Autodesk Inventor part; units mm, degrees
ref_plane "YZ Plane" through (0, 0, 0) normal (1, 0, 0) x (0, 1, 0)
ref_plane "XZ Plane" through (0, 0, 0) normal (0, 1, 0) x (-1, 0, 0)
ref_plane "XY Plane" through (0, 0, 0) normal (0, 0, 1) x (1, 0, 0)
sketch "Sketch1" plane through (0, 0, 0) normal (0, 0, 1) x (1, 0, 0)
  line L0 (0, 0) -> (225, 0)
  line L1 (225, 0) -> (225, 50)
  line L2 (225, 50) -> (0, 50)
  line L3 (0, 50) -> (0, 0)
  line L4 (-3, 45) -> (0, 45)
  line L5 (0, 45) -> (0, 38.75)
  line L6 (0, 38.75) -> (-3, 38.75)
  line L7 (-3, 38.75) -> (-3, 45)
  line L8 (0, 0) -> (15, 0)
  line L9 (15, 0) -> (15, -3)
  line L10 (15, -3) -> (0, -3)
  line L11 (0, -3) -> (0, 0)
  line L12 (-3, 33.75) -> (0, 33.75)
  line L13 (0, 33.75) -> (0, 27.5)
  line L14 (-3, 27.5) -> (-3, 33.75)
  line L15 (0, 27.5) -> (-3, 27.5)
  line L16 (-3, 22.5) -> (0, 22.5)
  line L17 (0, 22.5) -> (0, 16.25)
  line L18 (-3, 16.25) -> (-3, 22.5)
  line L19 (0, 16.25) -> (-3, 16.25)
  line L20 (-3, 11.25) -> (0, 11.25)
  line L21 (0, 11.25) -> (0, 5)
  line L22 (-3, 5) -> (-3, 11.25)
  line L23 (0, 5) -> (-3, 5)
  line L24 (225, 45) -> (228, 45)
  line L25 (228, 45) -> (228, 38.75)
  line L26 (225, 38.75) -> (225, 45)
  line L27 (228, 38.75) -> (225, 38.75)
  line L28 (225, 33.75) -> (228, 33.75)
  line L29 (228, 33.75) -> (228, 27.5)
  line L30 (225, 27.5) -> (225, 33.75)
  line L31 (228, 27.5) -> (225, 27.5)
  line L32 (225, 22.5) -> (228, 22.5)
  line L33 (228, 22.5) -> (228, 16.25)
  line L34 (225, 16.25) -> (225, 22.5)
  line L35 (228, 16.25) -> (225, 16.25)
  line L36 (225, 11.25) -> (228, 11.25)
  line L37 (228, 11.25) -> (228, 5)
  line L38 (225, 5) -> (225, 11.25)
  line L39 (228, 5) -> (225, 5)
  line L40 (45, -3) -> (30, -3)
  line L41 (30, -3) -> (30, 0)
  line L42 (45, 0) -> (45, -3)
  line L43 (30, 0) -> (45, 0)
  line L44 (75, -3) -> (60, -3)
  line L45 (60, -3) -> (60, 0)
  line L46 (75, 0) -> (75, -3)
  line L47 (60, 0) -> (75, 0)
  line L48 (105, -3) -> (90, -3)
  line L49 (90, -3) -> (90, 0)
  line L50 (105, 0) -> (105, -3)
  line L51 (90, 0) -> (105, 0)
  line L52 (135, -3) -> (120, -3)
  line L53 (120, -3) -> (120, 0)
  line L54 (135, 0) -> (135, -3)
  line L55 (120, 0) -> (135, 0)
  line L56 (165, -3) -> (150, -3)
  line L57 (150, -3) -> (150, 0)
  line L58 (165, 0) -> (165, -3)
  line L59 (150, 0) -> (165, 0)
  line L60 (195, -3) -> (180, -3)
  line L61 (180, -3) -> (180, 0)
  line L62 (195, 0) -> (195, -3)
  line L63 (180, 0) -> (195, 0)
  line L64 (225, -3) -> (210, -3)
  line L65 (210, -3) -> (210, 0)
  line L66 (225, 0) -> (225, -3)
  line L67 (210, 0) -> (225, 0)
  line L68 (15, 50) -> (0, 50)
  line L69 (0, 50) -> (0, 53)
  line L70 (15, 53) -> (15, 50)
  line L71 (0, 53) -> (15, 53)
  line L72 (45, 50) -> (30, 50)
  line L73 (30, 50) -> (30, 53)
  line L74 (45, 53) -> (45, 50)
  line L75 (30, 53) -> (45, 53)
  line L76 (75, 50) -> (60, 50)
  line L77 (60, 50) -> (60, 53)
  line L78 (75, 53) -> (75, 50)
  line L79 (60, 53) -> (75, 53)
  line L80 (105, 50) -> (90, 50)
  line L81 (90, 50) -> (90, 53)
  line L82 (105, 53) -> (105, 50)
  line L83 (90, 53) -> (105, 53)
  line L84 (135, 50) -> (120, 50)
  line L85 (120, 50) -> (120, 53)
  line L86 (135, 53) -> (135, 50)
  line L87 (120, 53) -> (135, 53)
  line L88 (165, 50) -> (150, 50)
  line L89 (150, 50) -> (150, 53)
  line L90 (165, 53) -> (165, 50)
  line L91 (150, 53) -> (165, 53)
  line L92 (195, 50) -> (180, 50)
  line L93 (180, 50) -> (180, 53)
  line L94 (195, 53) -> (195, 50)
  line L95 (180, 53) -> (195, 53)
  line L96 (225, 50) -> (210, 50)
  line L97 (210, 50) -> (210, 53)
  line L98 (225, 53) -> (225, 50)
  line L99 (210, 53) -> (225, 53)
  point P0 (0, 38.75)
  point P1 (0, 50)
  dimension "d0" = 225
  dimension "d1" = 50
  dimension "d4" = 6.25
  dimension "d5" = 3
  dimension "d6" = 5
  dimension "d7" = 15
  dimension "d8" = 3
  dimension "d13" = 11.25
  dimension "d16" = 228
  dimension "d21" = 30
  dimension "d24" = 53
extrude "Extrusion1" add sketch "Sketch1" along normal blind 3 contours L3 L2 L1 L0 | L23 L22 L20 L3 | L19 L18 L16 L3 | L15 L14 L12 L3 | L6 L7 L4 L3 | L1 L36 L37 L39 | L1 L32 L33 L35 | L1 L28 L29 L31 | L1 L24 L25 L27
extrude "Extrusion2" add sketch "Sketch1" along normal blind 3 contours L0 L9 L10 L11 | L0 L42 L40 L41 | L0 L46 L44 L45 | L0 L50 L48 L49 | L0 L54 L52 L53 | L69 L71 L70 L2 | L0 L58 L56 L57 | L73 L75 L74 L2 | L0 L62 L60 L61 | L77 L79 L78 L2 | L0 L66 L64 L65 | L81 L83 L82 L2 | L85 L87 L86 L2 | L89 L91 L90 L2 | L93 L95 L94 L2 | L97 L99 L98 L2
properties part number "AnchoBase"
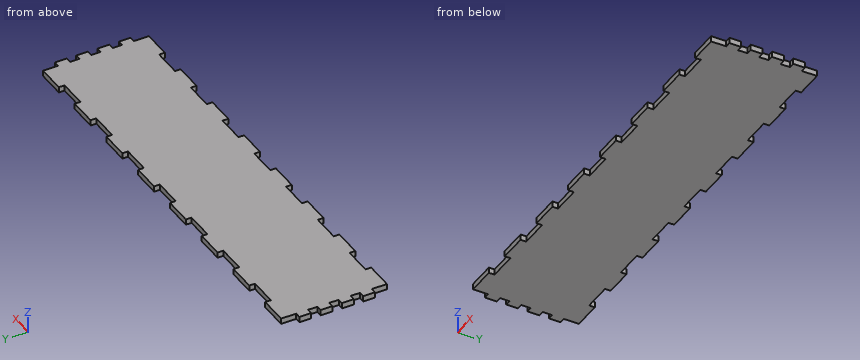
The listing builds one solid part. Answer for the finished solid, in the listing's coordinates (mm). Coordinates: 2 decimals unless noted, no trailing zeros. Loops run counter-clockwise (first coordinate to the right, second up) from the corner with the lowest first, then second, coordinate; pieces in that order, holes last.
1) Find the intervals of material crossed by L1, parallel to X at y = 23.5, z = 0.45; L2, parallel to Y at x = 199, z = 0.2, in increasing order.
2) Flat-ended cylindrical pins translate along their axes: pin 1 Ø0.9 at (x, z) = (113.5, 1) entering from -Y; pin 2 Ø1.5 at (y, z) = (52, 2) entering from -X; pin 3 Ø1.5 at (y, z) = (25, 2) entering from +X; pin 4 Ø1.5 at (x, z) = (105.5, 2) entering from -Y. Find the tip coordinate at first contact, or state that the pin passes through.
3) Find section A-A on y = 3. Write down the section's boundary in (x, z), then the cut area to 3 significant figures.
4) Find section B-B on x = 167. Write down the section's boundary in (y, z), then the cut area to 3 significant figures.
Values:
1. L1: x = 0 to 225
1. L2: y = 0 to 50
2. pin 1: stops at y = 0
2. pin 2: stops at x = 0
2. pin 3: stops at x = 225
2. pin 4: stops at y = -3
3. outline: (0, 0) - (225, 0) - (225, 3) - (0, 3) - close
3. area: 675 mm2
4. outline: (0, 0) - (50, 0) - (50, 3) - (0, 3) - close
4. area: 150 mm2
